Autodesk Inventor part; units mm, degrees
ref_plane "YZ Plane" through (0, 0, 0) normal (1, 0, 0) x (0, 1, 0)
ref_plane "XZ Plane" through (0, 0, 0) normal (0, 1, 0) x (-1, 0, 0)
sketch "Sketch1" plane through (0, 0, 0) normal (0, 0, 1) x (1, 0, 0)
  line L0 (-3.175, 3.175) -> (3.175, 3.175)
  line L1 (3.175, 3.175) -> (3.175, -3.175)
  line L2 (3.175, -3.175) -> (-3.175, -3.175)
  line L3 (-3.175, -3.175) -> (-3.175, 3.175)
  line L4 (-3.175, 3.175) -> (3.175, -3.175) construction
  line L5 (3.175, 3.175) -> (-3.175, -3.175) construction
  point P0 (0, 0)
  dimension "d0" = 6.35
  dimension "d1" = 6.35
extrude "Extrusion1" add sketch "Sketch1" along normal blind 1
sketch "Sketch2" plane through (0, 0, 1) normal (0, 0, 1) x (1, 0, 0)
  circle A0 centre (-1.905, -1.905) radius 0.325
  line L0 (-3.175, 3.175) -> (-3.175, -3.175)
  line L1 (-3.175, -3.175) -> (3.175, -3.175)
  point P0 (0, 0)
  dimension "d4" = 0.65
  dimension "d5" = 1.27
  dimension "d6" = 1.27
extrude "Extrusion2" cut sketch "Sketch2" against normal through all
sketch "Sketch3" plane through (0, 0, 1) normal (0, 0, 1) x (1, 0, 0)
  circle A0 centre (-1.905, -1.905) radius 0.325
  circle A1 centre (-1.905, -1.905) radius 0.5
  point P0 (0, 0)
  dimension "d15" = 1
extrude "Extrusion3" add sketch "Sketch3" along normal blind 0.015
ref_plane "Work Plane1" through (0, 0, 0.5) normal (0, 0, 1) x (1, 0, 0)
pattern_linear "Rectangular Pattern3" count 4 spacing 1.27 along (1, 0, 0) count 4 spacing 1.27 along (0, 1, 0) of "Extrusion2"
pattern_linear "Rectangular Pattern4" count 4 spacing 1.27 along (1, 0, 0) count 4 spacing 1.27 along (0, 1, 0) of "Extrusion3"
mirror "Mirror2" about plane through (0, 0, 0.5) normal (0, 0, 1) of "Extrusion3", "Rectangular Pattern4"
equation "\"BendRadius\" = Thickness"
equation "\"BendReliefWidth\" = Thickness"
equation "\"BendReliefDepth\" = 0.5 * Thickness"
equation "\"CornerReliefSize\" = 4 * Thickness"
equation "\"MinimumRemnant\" = 2 * Thickness"
equation "\"TransitionRadius\" = BendRadius"
equation "\"JacobiRadiusSize\" = BendRadius"
equation "\"GapSize\" = Thickness"
properties part number "1.27mmpitchProtoboardDesign.ipt_.25inch_.25Inch"
For this review, take the finished solid that the model builds, in its own axes (mm). Round coordinates to 2 decimals unless told otherwise and drop trailing zeros. Write each loop counter-clockwise with the first axis right and the second up, starting at its lowest first coordinate (ties: lowest second). Pieces come first, ordered by that corner, then holes. Notation, with made-up numbers: (-33.5, -9) - (-27.5, -9) arc R17 cw to (-27.5, 15) - close; hole circle Ø6 at (-20, 85.5). An arc over 180 degrees is marked (long way). Answer as CSV lines item,"result". Start each with the question number.
(1) For line 1 (X direction, y = 1.75, z = 0.55) (3 decimals); line 2 (Y direction, x = -0.75, z = 0.45) (3 decimals); line 3 (Z direction, x = 3, y = -1.75), list the stretches that pass through material, from the lowest coordinate up.
(2) Add section A-A, the plane z = 0.35. State how many separate pieces and enclosed holes the cut face has, plus the area to 3 significant figures.
(3) Add section C-C, the plane x = 0. State the section outline as (y, z) points (3 decimals).
From the geometry:
1,line 1,"x = -3.175 to -2.191, -1.619 to -0.921, -0.349 to 0.349, 0.921 to 1.619, 2.191 to 3.175"
1,line 2,"y = -3.175 to -2.209, -1.601 to -0.939, -0.331 to 0.331, 0.939 to 1.601, 2.209 to 3.175"
1,line 3,"z = 0 to 1"
2,separate pieces,"1"
2,enclosed holes,"16"
2,area,"35.0 mm²"
3,outline,"(-3.175, 0) - (3.175, 0) - (3.175, 1) - (-3.175, 1) - close"
